```python
from build123d import *

# Parameters (mm, degrees)
BOSS_EXTRUDE1_DEPTH = 76.2
SKETCH2_R           = 2.4892
CUT_EXTRUDE1_DEPTH  = 4.175


with BuildPart() as part:
    # Sketch1 → Boss-Extrude1 (new body, symmetric)
    with BuildSketch(Plane.XY):
        Polygon((0, 9.525), (0, 0), (25.4, 0), (25.4, 3.175), (3.175, 3.175), (3.175, 9.525), align=None)
    extrude(amount=BOSS_EXTRUDE1_DEPTH, both=True)

    # Sketch2 → Cut-Extrude1 (cut, through all)
    with BuildSketch(Plane(origin=(0, 3.175, 0), x_dir=(1, 0, 0), z_dir=(0, 1, 0))):
        with Locations((12.7, -63.5)):
            Circle(SKETCH2_R)
        with Locations((12.7, 63.5)):
            Circle(SKETCH2_R)
    extrude(amount=-CUT_EXTRUDE1_DEPTH, mode=Mode.SUBTRACT)


solid = part.part
```
The model under review builds one solid part; all positions refer to its coordinate system, in mm. A direction names the side the tool comes from. Give positions to 0.01 mm unless a question says otherwise; leave off trailing zeros. Write each loop counter-clockwise with the first axis right and the second up, starting at its lowest first coordinate (ties: lowest second). Pieces come first, ordered by that corner, then holes. Notation, with made-up numbers: (89, -33) -> (141, -33) arc R7 cw to (141, -20) -> close; hole circle Ø9 at (-11, 62.25). An arc over 180 degrees is marked (long way). Answer in a Markdown table with one row per item.
1) Tool access review of faces 4 (the flat face through (10, 3, -76.2)), 5 (the flat face through (3.175, 6, 1)): name each direction out of +Z, -Z, +X, -X, +Y, -Y from which nothing blocks a thin tool from reaching the whole face with its end or side.
Worked answers:
| item | result |
|---|---|
| face 4 | -Z, +X, -X, +Y, -Y |
| face 5 | +Z, -Z, +X, +Y |
2) Add section C-C on x = 19.5. State the section outline as (y, z) points (3 decimals).
Worked answers:
| item | result |
|---|---|
| outline | (0, -76.2) -> (3.175, -76.2) -> (3.175, 76.2) -> (0, 76.2) -> close |
3) Add section B-B on x = 12.7. State the section outline as (y, z) points (3 decimals), plus the area to 3 significant figures.
Worked answers:
| item | result |
|---|---|
| outline | (0, -76.2) -> (3.175, -76.2) -> (3.175, -65.989) -> (0, -65.989) -> close; (0, -61.011) -> (3.175, -61.011) -> (3.175, 61.011) -> (0, 61.011) -> close; (0, 65.989) -> (3.175, 65.989) -> (3.175, 76.2) -> (0, 76.2) -> close |
| area | 452 mm² |
4) For L1, parallel to Z at x = 12.7, y = 1.5; L2, parallel to X at y = 1.85, z = -63.5; L3, parallel to X at y = 5.5, z = 54.5 (3 decimals), list the stretches that pass through material, from the lowest coordinate up. Write a range as [from, to].
Worked answers:
| item | result |
|---|---|
| L1 | [-76.2, -65.99], [-61.01, 61.01], [65.99, 76.2] |
| L2 | [0, 10.21], [15.19, 25.4] |
| L3 | [0, 3.175] |
5) Clearance check with flat-ended pins moving along their axes: P1, Ø1.5, axis at y = 4, z = 23, coming from the +X side (3 decimals); P2, Ø5, axis at x = 10.5, z = 55, coming from the +Y side (3 decimals). State where each tip first meets the part, or that it passes through.
Worked answers:
| item | result |
|---|---|
| P1 | x = 3.175 |
| P2 | y = 3.175 |
6) Add section A-A on z = -63.5. State the section outline as (x, y) points (3 decimals).
Worked answers:
| item | result |
|---|---|
| outline | (0, 0) -> (10.211, 0) -> (10.211, 3.175) -> (3.175, 3.175) -> (3.175, 9.525) -> (0, 9.525) -> close; (15.189, 0) -> (25.4, 0) -> (25.4, 3.175) -> (15.189, 3.175) -> close |
7) Mouldability with a two-part tool opening along X and no side actions: class faces 1 (the cylindrical face through (14.04, 1.61, -65.6)), 2 (the flat face through (25.4, 2, 1)), 3 (the flat face through (0, 5, 1)) as +X half, -X half, draft (parallel to the pull), parting line (faces both ways), or undercut.
Worked answers:
| item | result |
|---|---|
| face 1 | undercut |
| face 2 | +X half |
| face 3 | -X half |
